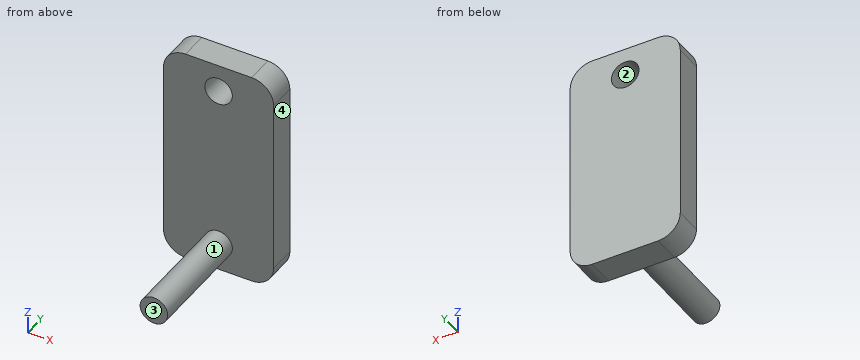
from build123d import *

# Parameters (mm, degrees)
F0_W     = 25.4
F0_H     = 50.8
F0_R     = 3.175
F1_DEPTH = 6.35
F2_R     = 5.08
F3_R     = 5.08
F4_R     = 5.08
F5_R     = 3.175
F6_DEPTH = 25.4


with BuildPart() as f1:
    # F0 (on Front) → F1 (new body)
    with BuildSketch(Plane.XZ):
        with Locations((12.7, -25.4)):
            Rectangle(F0_W, F0_H)
        with Locations((12.7, -6.35)):
            Circle(F0_R, mode=Mode.SUBTRACT)
    extrude(amount=F1_DEPTH)

    # F2
    f2_edges = [f1.edges().sort_by_distance(p)[0] for p in [
        (0, -3.175, 0),
    ]]
    fillet(f2_edges, radius=F2_R)

    # F3
    f3_edges = [f1.edges().sort_by_distance(p)[0] for p in [
        (25.4, -3.175, 0),
    ]]
    fillet(f3_edges, radius=F3_R)

    # F4
    f4_edges = [f1.edges().sort_by_distance(p)[0] for p in [
        (25.4, -3.175, -50.8),
        (0, -3.175, -50.8),
    ]]
    fillet(f4_edges, radius=F4_R)

    # F5 (on face) → F6 (join)
    with BuildSketch(Plane.XZ.offset(6.35)):
        with Locations((12.7, -44.45)):
            Circle(F5_R)
    extrude(amount=F6_DEPTH)


solid = f1.part
Here's how the part is built. I have some questions about the finished solid (model axes, mm). Face numbers are marked on the shaded views. Give positions to 0.01 mm unless a question says otherwise; leave off trailing zeros. Order: outer loops, then holes, each group sorted by start corner. A loop starts at its lowest first (then second) coordinate and runs counter-clockwise, first axis right, second up. Notation, with made-up numbers: (68, 35.25) -> (99, 35.25) arc R34 cw to (99, 66.25) -> close; hole circle Ø9 at (24, -25.75). An arc over 180 degrees is marked (long way). One line per item, written item: value. Start each with the question number.
1. Imagine slicing it at A-A, the plane z = -6.35. List the corners of the cut face in (x, y) for me (3 decimals).
2. Imagine slicing it at B-B, the plane y = -3.5. List the corners of the cut face in (x, z) for me (3 decimals), plus the area to 3 significant figures.
3. I need wall thicknesses on probe 1 along Z at (x, y) = (12.7, -4.5) (3 decimals); probe 2 along Y at (x, z) = (16.5, -19); probe 3 along X at (y, z) = (-4, -6). Which ranges of each line are inside material? Lowest first, please. Write a range as from..to.
4. Will these pins go through, and if not, where does the flat tip stop? pin 1 Ø3 at (x, z) = (6, -7.5) entering from -Y; pin 2 Ø3 at (x, y) = (11.5, -10.5) entering from +Z (3 decimals); pin 3 Ø5 at (x, y) = (17.5, -10.5) entering from +Z.
5. We'd pull the mould along X, two halves only. Please class the marked faces 1, 2, 3 and 4: released by +X, released by -X, zero draft, split by the parting line, or undercut.
6. Imagine slicing it at C-C, the plane x = 12.7. List the corners of the cut face in (y, z) for me (3 decimals), plus the area to 3 significant figures.
7. Imagine slicing it at D-D, the plane z = -44.45. List the corners of the cut face in (x, y) for me (3 decimals).
Values follow:
1. outline: (0, -6.35) -> (9.525, -6.35) -> (9.525, 0) -> (0, 0) -> close; (15.875, -6.35) -> (25.4, -6.35) -> (25.4, 0) -> (15.875, 0) -> close
2. outline: (0, -45.72) arc R5.08 ccw to (5.08, -50.8) -> (20.32, -50.8) arc R5.08 ccw to (25.4, -45.72) -> (25.4, -5.08) arc R5.08 ccw to (20.32, 0) -> (5.08, 0) arc R5.08 ccw to (0, -5.08) -> close; hole circle Ø6.35 at (12.7, -6.35)
2. area: 1,240 mm2
3. probe 1: z = -50.8..-9.525, -3.175..0
3. probe 2: y = -6.35..0
3. probe 3: x = 0..9.54, 15.86..25.4
4. pin 1: stops at y = -6.35
4. pin 2: stops at z = -41.275
4. pin 3: stops at z = -42.26
5. face 1: split by the parting line
5. face 2: undercut
5. face 3: zero draft
5. face 4: released by +X
6. outline: (-31.75, -47.625) -> (-6.35, -47.625) -> (-6.35, -50.8) -> (0, -50.8) -> (0, -9.525) -> (-6.35, -9.525) -> (-6.35, -41.275) -> (-31.75, -41.275) -> close; (-6.35, -3.175) -> (0, -3.175) -> (0, 0) -> (-6.35, 0) -> close
6. area: 444 mm2
7. outline: (0, -6.35) -> (9.525, -6.35) -> (9.525, -31.75) -> (15.875, -31.75) -> (15.875, -6.35) -> (25.4, -6.35) -> (25.4, 0) -> (0, 0) -> close
